from build123d import *

# Parameters (mm, degrees)
F0_R     = 11
F0_R_2   = 4
F1_DEPTH = 2.5
F0_R_3   = 3.9
F2_DEPTH = 0.8
F5_R     = 5
F5_R_2   = 4
F6_DEPTH = 1


with BuildPart() as f1:
    # F0 (on Top) → F1 (new body)
    with BuildSketch(Plane.XY):
        Circle(F0_R)
        Circle(F0_R_2, mode=Mode.SUBTRACT)
    extrude(amount=F1_DEPTH)

    # F0 (on Top) → F2 (join)
    with BuildSketch(Plane.XY):
        Circle(F0_R_2)
        Circle(F0_R_3, mode=Mode.SUBTRACT)
        Circle(F0_R_3)
    extrude(amount=F2_DEPTH)

    # F3 (on Front) → F4 (revolve, cut)
    with BuildSketch(Plane.XZ):
        with BuildLine():
            add(Edge.make_bspline(
                [(4, 2.5), (4.80237, 2.181631), (5.20459, 1.426604), (4.788445, 0.966279), (4, 0.5)],
                knots=[0, 0, 0, 0, 1.41393, 2.828427, 2.828427, 2.828427, 2.828427], degree=3))
            Line((4, 2.5), (4, 0.5))
        make_face()
    revolve(axis=Axis((0, 0, 1.641661), (0, 0, 1)), mode=Mode.SUBTRACT)

    # F5 (on face) + F0 (on Top) → F6 (join)
    with BuildSketch(Plane.XY.offset(2.5)):
        Circle(F5_R)
        Circle(F5_R_2, mode=Mode.SUBTRACT)
    with BuildSketch(Plane.XY):
        Circle(F0_R)
        Circle(F0_R_2, mode=Mode.SUBTRACT)
    extrude(amount=F6_DEPTH)


solid = f1.part
CAD build for the part. Positions are in the model's coordinates, mm. A direction names the side the tool comes from. Round coordinates to 2 decimals unless told otherwise and drop trailing zeros. Write each loop counter-clockwise with the first axis right and the second up, starting at its lowest first coordinate (ties: lowest second). Pieces come first, ordered by that corner, then holes. Notation, with made-up numbers: M 87,3.25 L 95,3.25 A9 ccw 95,7.25 Z; hole C 62.25,69.5 d6. An arc over 180 degrees is marked long. Use a Markdown table: item, result. Add a question column.
1. Slice it at C-C on x = -6.5. Give the cut face in (y, z), then the cut area to 3 significant figures.
2. Drill centre lines: probe 1 along Y at (x, z) = (0, 2.9); probe 2 along Z at (x, y) = (-5.5, 6.5); probe 3 along Y at (x, z) = (0, 0.9). Where is each one in solid material? Low to high.
3. Pull direction X, two halves, no side cores. Call faces 3 (the face through (0, 0, 0)), 4 (the face through (-1.08, -4.88, 2.99)), 5 (the face through (-4, -2, 1)): released by +X, released by -X, zero draft, split by the parting line, or undercut.
4. Slice it at A-A on z = 3. Give the cut face in (x, y).
5. 3-axis set-ups, long thin cutter, end or side, ignore diameter. For faces 1 (the face through (-0.867, -3.905, 2.993)), 2 (the face through (-2.38, -10.74, 1.23)): which of +Z, -Z, +X, -X, +Y, -Y reach the whole face in a straight line?
6. Slice it at B-B on z = 0.3. Give the cut face in (x, y).
7. Flat gauge pins, fed straight in: P1, Ø12, axis at x = 8.5, y = -7.5, coming from the +Z side; P2, Ø7, axis at x = 0, y = 0, coming from the +Z side; P3, Ø2, axis at y = -5, z = 0.5, coming from the +X side. Where does each tip first touch, or does it go through?
Reply:
| question | item | result |
|---|---|---|
| 1 | outline | M -8.87,0 L 8.87,0 L 8.87,2.5 L -8.87,2.5 Z |
| 1 | area | 44.4 mm^2 |
| 2 | probe 1 | y = -5 to -4, 4 to 5 |
| 2 | probe 2 | z = 0 to 2.5 |
| 2 | probe 3 | y = -11 to -4, 4 to 11 |
| 3 | face 3 | zero draft |
| 3 | face 4 | split by the parting line |
| 3 | face 5 | undercut |
| 4 | outline | C 0,0 d10; hole C 0,0 d8 |
| 5 | face 1 | +Z |
| 5 | face 2 | +Z, -Z |
| 6 | outline | C 0,0 d22 |
| 7 | P1 | stops at z = 2.5 |
| 7 | P2 | stops at z = 0.8 |
| 7 | P3 | stops at x = 10.25 |
